Geometry check sheet. Reference: drawing and pictorial views, mm from the part's lowest x, y, z. Give positions to 0.01 mm unless a question says otherwise; leave off trailing zeros. Write each loop counter-clockwise with the first axis right and the second up, starting at its lowest first coordinate (ties: lowest second). Pieces come first, ordered by that corner, then holes. Notation, with made-up numbers: (79, 38) - (124, 38) arc R35 cw to (124, 76) - close; hole circle Ø1 at (76.25, 56.5). An arc over 180 degrees is marked (long way). Put each result on its own line as item: value.
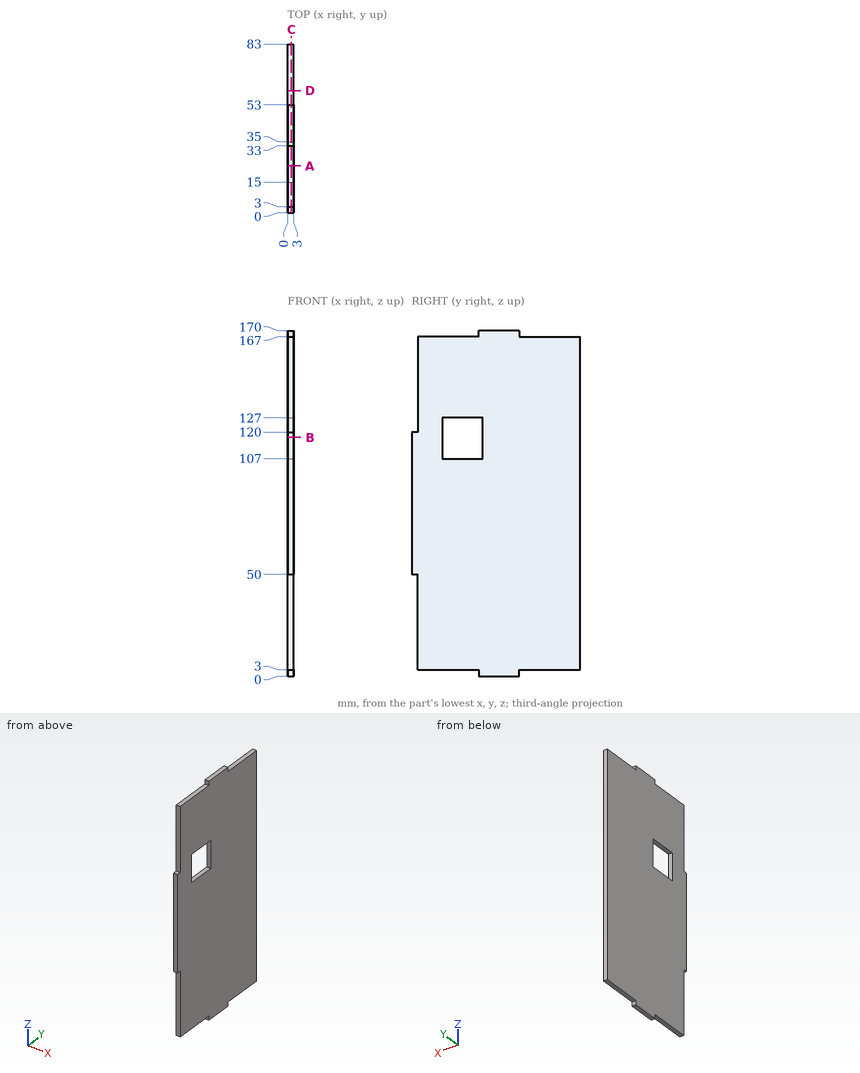
Q1. Section check B-B, the plane z = 117.5. Record the cut outline in (x, y), plus the area to 3 significant figures.
Answers follow:
outline: (0, 0) - (3, 0) - (3, 15) - (0, 15) - close; (0, 35) - (3, 35) - (3, 83) - (0, 83) - close
area: 189 mm2
Q2. Scan lines: line 1 along Y through (x, z) = (2.8, 139); line 2 along Y through (x, z) = (0.45, 122.5); line 3 along Z through (x, y) = (1.75, 64). Record each from-to range of solid material in increasing order.
Answers follow:
line 1: y = 3 to 83
line 2: y = 3 to 15, 35 to 83
line 3: z = 3 to 167
Q3. Section check C-C, the plane x = 1.85. Record the cut outline in (y, z), plus the area to 4 significant figures.
Answers follow:
outline: (0, 50) - (3, 50) - (3, 3) - (33, 3) - (33, 0) - (53, 0) - (53, 3) - (83, 3) - (83, 167) - (53, 167) - (53, 170) - (33, 170) - (33, 167) - (3, 167) - (3, 120) - (0, 120) - close; hole (15, 107) - (35, 107) - (35, 127) - (15, 127) - close
area: 13,050 mm2
Q4. Section check A-A, the plane y = 23. Record the cut outline in (x, z).
Answers follow:
outline: (0, 3) - (3, 3) - (3, 107) - (0, 107) - close; (0, 127) - (3, 127) - (3, 167) - (0, 167) - close
Q5. Section check D-D, the plane y = 60. Record the cut outline in (x, z).
Answers follow:
outline: (0, 3) - (3, 3) - (3, 167) - (0, 167) - close
Q6. Go/stop test with flat-tipped pins: pin 1 Ø1.5 at (x, z) = (2, 32) entering from -Y; pin 2 Ø0.9 at (x, y) = (2, 13) entering from +Z; pin 3 Ø1.5 at (x, z) = (2, 168) entering from -Y. Record where each tip stops, or that it passes through.
Answers follow:
pin 1: stops at y = 3
pin 2: stops at z = 167
pin 3: stops at y = 33
